```python
from build123d import *

# Parameters (mm, degrees)
OUTER_FLANGE_CONTACT_ANNULUS_ID8P2_START = -3
SKETCH1_R                                = 8
SKETCH1_R_2                              = 4.1
OUTER_FLANGE_CONTACT_ANNULUS_ID8P2_DEPTH = 0.5
M14X0P5_INTERNAL_THREAD_ENVELOPE_START   = -2.5
SKETCH2_R                                = 8
SKETCH2_R_2                              = 7
M14X0P5_INTERNAL_THREAD_ENVELOPE_DEPTH   = 1.2
SKETCH3_R                                = 0.6
TWO_PIN_WRENCH_HOLES_D1P2_DEPTH          = 0.5001


with BuildPart() as part:
    # Sketch1 → Outer_Flange_Contact_Annulus_ID8p2 (new body)
    with BuildSketch(Plane.XY.offset(OUTER_FLANGE_CONTACT_ANNULUS_ID8P2_START)):
        Circle(SKETCH1_R)
        Circle(SKETCH1_R_2, mode=Mode.SUBTRACT)
    extrude(amount=OUTER_FLANGE_CONTACT_ANNULUS_ID8P2_DEPTH)

    # Sketch2 → M14x0p5_Internal_Thread_Envelope (add)
    with BuildSketch(Plane.XY.offset(M14X0P5_INTERNAL_THREAD_ENVELOPE_START)):
        Circle(SKETCH2_R)
        Circle(SKETCH2_R_2, mode=Mode.SUBTRACT)
    extrude(amount=M14X0P5_INTERNAL_THREAD_ENVELOPE_DEPTH)

    # Sketch3 → Two_Pin_Wrench_Holes_D1p2 (cut)
    with BuildSketch(Plane(origin=(0, 0, -3), x_dir=(-1, 0, 0), z_dir=(0, 0, -1))):
        with Locations((7.1, 0)):
            Circle(SKETCH3_R)
        with Locations((-7.1, 0)):
            Circle(SKETCH3_R)
    extrude(amount=-TWO_PIN_WRENCH_HOLES_D1P2_DEPTH, mode=Mode.SUBTRACT)


solid = part.part
```
Read the model definition and answer for the solid it produces. Units are mm, in the model's axes. A direction names the side the tool comes from. Give positions to 0.01 mm unless a question says otherwise; leave off trailing zeros. Write each loop counter-clockwise with the first axis right and the second up, starting at its lowest first coordinate (ties: lowest second). Pieces come first, ordered by that corner, then holes. Notation, with made-up numbers: M 39.5,75 L 84.5,75 A7 ccw 84.5,88 Z; hole C -37,74.25 d9. An arc over 180 degrees is marked long. Put each result on its own line as item: value. Start each with the question number.
1. The part is cut by section D-D, the plane z = -1.85. Give the vertices of the cut face in (x, y), and give its area (3 significant figures).
2. For a pull along Y with two mould halves and no side action, classify faces 4 (the cylindrical face through (6.466, -2.681, -1.908)), 5 (the flat face through (4, -6, -1.3)), 6 (the cylindrical face through (-1.73, -7.81, -2.16)), 7 (the cylindrical face through (6.528, 0.18, -2.753)) as released by +Y, released by -Y, zero draft, split by the parting line, or undercut.
3. Which of the six approach directions +Z, -Z, +X, -X, +Y, -Y give full straight-line access (tool end or side, diameter ignored) to faces 1 (the flat face through (-4, 2, -3)), 2 (the flat face through (3.003, -3.013, -2.5)), 3 (the cylindrical face through (-7.672, 0.18, -2.753))?
4. The part is cut by section C-C, the plane y = -3. Give the vertices of the cut face in (x, z), and give its area (3 significant figures).
5. Each of these flat-tipped pins is pushed along its axis until it touches: pin 1 Ø1 at (x, z) = (-3, -1.5) entering from +Y; pin 2 Ø9.5 at (x, y) = (0, 0) entering from +Z. Where does it stop, or does it pass through?
6. The part is cut by section A-A, the plane x = 0. Give the vertices of the cut face in (y, z).
7. The part is cut by section B-B, the plane y = 0. Give the vertices of the cut face in (x, z), and give its area (3 significant figures).
8. Consider line 1 along Y through (x, z) = (0, -2.8); line 2 along Z through (x, y) = (-4, -3); line 3 along X through (y, z) = (4.25, -2.15). Determine where each line is inside the solid, lowest interval first.
Final values:
1. outline: C 0,0 d16; hole C 0,0 d14
1. area: 47.1 mm²
2. face 4: undercut
2. face 5: zero draft
2. face 6: split by the parting line
2. face 7: undercut
3. face 1: -Z, +X, -X, +Y, -Y
3. face 2: +Z
3. face 3: -Z
4. outline: M -7.42,-3 L -2.79,-3 L -2.79,-2.5 L -6.32,-2.5 L -6.32,-1.3 L -7.42,-1.3 Z; M 2.79,-3 L 7.42,-3 L 7.42,-1.3 L 6.32,-1.3 L 6.32,-2.5 L 2.79,-2.5 Z
4. area: 7.24 mm²
5. pin 1: stops at y = 7.6
5. pin 2: stops at z = -2.5
6. outline: M -8,-3 L -4.1,-3 L -4.1,-2.5 L -7,-2.5 L -7,-1.3 L -8,-1.3 Z; M 4.1,-3 L 8,-3 L 8,-1.3 L 7,-1.3 L 7,-2.5 L 4.1,-2.5 Z
7. outline: M -8,-3 L -7.7,-3 L -7.7,-2.5 L -7,-2.5 L -7,-1.3 L -8,-1.3 Z; M -6.5,-3 L -4.1,-3 L -4.1,-2.5 L -6.5,-2.5 Z; M 4.1,-3 L 6.5,-3 L 6.5,-2.5 L 4.1,-2.5 Z; M 7,-2.5 L 7.7,-2.5 L 7.7,-3 L 8,-3 L 8,-1.3 L 7,-1.3 Z
7. area: 5.10 mm²
8. line 1: y = -8 to -4.1, 4.1 to 8
8. line 2: z = -3 to -2.5
8. line 3: x = -6.78 to -5.56, 5.56 to 6.78
